from build123d import *

# Parameters (mm, degrees)
SKETCH41_R                  = 2.5527
BACK_PLATE_EXTRUDE_DEPTH    = 3.175
SKETCH71_W                  = 8.89
SKETCH71_H                  = 4.7625
SKETCH71_W_2                = 13.79855
SKETCH71_W_3                = 15.09395
BOSS_EXTRUDE26_DEPTH        = 3.175
SKETCH91_W                  = 4.9022
SKETCH91_H                  = 20.7645
SKETCH91_W_2                = 12.8524
SKETCH91_H_2                = 4.7625
SKETCH91_W_3                = 49.3649
SKETCH91_W_4                = 12.7762
BACK_PLATE_TOLERENCES_DEPTH = 4.175
SKETCH92_W                  = 2.794
SKETCH92_H                  = 26.9875
CUT_EXTRUDE1_DEPTH          = 4.175
FILLET27_R                  = 0.635
FILLET28_R                  = 0.635
SKETCH93_R                  = 0.635
CUT_EXTRUDE2_DEPTH          = 4.175
FILLET29_R                  = 0.635
FILLET29_OF_MIRROR26_R      = 0.635


with BuildPart() as part:
    # Sketch41 → Back Plate Extrude------------ (new body)
    with BuildSketch(Plane.XY.offset(152.527)):
        Polygon((-104.775, -7.9375), (-104.775, 12.7), (-109.5248, 12.7), (-109.5248, 3.175), (-112.395, 3.175), (-112.395, 25.4), (-104.775, 25.4), (104.775, 25.4), (112.395, 25.4), (112.395, 3.175), (109.5248, 3.175), (109.5248, 12.7), (104.775, 12.7), (104.775, -7.9375), align=None)
        with Locations((-100.0125, 3.9624)):
            Circle(SKETCH41_R, mode=Mode.SUBTRACT)
        with Locations((100.0125, 3.9624)):
            Circle(SKETCH41_R, mode=Mode.SUBTRACT)
        with Locations((23.8252, 20.6375)):
            Circle(SKETCH41_R, mode=Mode.SUBTRACT)
        with Locations((38.1127, 20.6375)):
            Circle(SKETCH41_R, mode=Mode.SUBTRACT)
        with Locations((52.4002, 20.6375)):
            Circle(SKETCH41_R, mode=Mode.SUBTRACT)
        with Locations((66.6877, 20.6375)):
            Circle(SKETCH41_R, mode=Mode.SUBTRACT)
        with Locations((-66.6877, 20.6375)):
            Circle(SKETCH41_R, mode=Mode.SUBTRACT)
        with Locations((-52.4002, 20.6375)):
            Circle(SKETCH41_R, mode=Mode.SUBTRACT)
        with Locations((-38.1127, 20.6375)):
            Circle(SKETCH41_R, mode=Mode.SUBTRACT)
        with Locations((-23.8252, 20.6375)):
            Circle(SKETCH41_R, mode=Mode.SUBTRACT)
        with Locations((-87.3125, 3.9624)):
            Circle(SKETCH41_R, mode=Mode.SUBTRACT)
        with Locations((87.3125, 3.9624)):
            Circle(SKETCH41_R, mode=Mode.SUBTRACT)
        with Locations((-63.5, -1.5875)):
            Circle(SKETCH41_R, mode=Mode.SUBTRACT)
        with Locations((63.5, -1.5875)):
            Circle(SKETCH41_R, mode=Mode.SUBTRACT)
    extrude(amount=BACK_PLATE_EXTRUDE_DEPTH)

    # Sketch71 → Boss-Extrude26 (add, through all)
    with BuildSketch(Plane.XY.offset(155.702)):
        with Locations((-107.95, 27.78125)):
            Rectangle(SKETCH71_W, SKETCH71_H)
        with Locations((-83.905725, 27.78125)):
            Rectangle(SKETCH71_W_2, SKETCH71_H)
        with Locations((-20.246975, 27.78125)):
            Rectangle(SKETCH71_W_3, SKETCH71_H)
    boss_extrude26 = extrude(amount=-BOSS_EXTRUDE26_DEPTH)

    # Mirror23: Boss-Extrude26 across plane
    add(boss_extrude26.mirror(Plane(origin=(0, 0, 0), x_dir=(0, 0, 1), z_dir=(1, 0, 0))))

    # Sketch91 → Back Plate Tolerences (cut, through all)
    with BuildSketch(Plane(origin=(0, 0, 152.527), x_dir=(-1, 0, 0), z_dir=(0, 0, -1))):
        with Locations((-107.1499, 2.44475)):
            Rectangle(SKETCH91_W, SKETCH91_H)
        with Locations((-97.155, 27.78125)):
            Rectangle(SKETCH91_W_2, SKETCH91_H_2)
        with Locations((-52.4002, 27.78125)):
            Rectangle(SKETCH91_W_3, SKETCH91_H_2)
        with Locations((-6.3881, 27.78125)):
            Rectangle(SKETCH91_W_4, SKETCH91_H_2)
    back_plate_tolerences = extrude(amount=-BACK_PLATE_TOLERENCES_DEPTH, mode=Mode.SUBTRACT)

    # Mirror25: Back Plate Tolerences across plane
    add(back_plate_tolerences.mirror(Plane(origin=(0, 0, 0), x_dir=(0, 0, 1), z_dir=(1, 0, 0))), mode=Mode.SUBTRACT)

    # Sketch92 → Cut-Extrude1 (cut, through all)
    with BuildSketch(Plane.XY.offset(155.702)):
        with Locations((-110.998, 16.66875)):
            Rectangle(SKETCH92_W, SKETCH92_H)
        with Locations((110.998, 16.66875)):
            Rectangle(SKETCH92_W, SKETCH92_H)
    extrude(amount=-CUT_EXTRUDE1_DEPTH, mode=Mode.SUBTRACT)

    # Fillet27
    fillet27_edges = [part.edges().sort_by_distance(p)[0] for p in [
        (104.6988, -7.9375, 154.1145),
        (109.601, 12.827, 154.1145),
        (-109.601, 12.827, 154.1145),
        (-104.6988, -7.9375, 154.1145),
        (-109.601, 30.1625, 154.1145),
        (109.601, 30.1625, 154.1145),
    ]]
    fillet(fillet27_edges, radius=FILLET27_R)

    # Fillet28
    fillet28_edges = [part.edges().sort_by_distance(p)[0] for p in [
        (103.5812, 30.1625, 154.1145),
        (90.7288, 30.1625, 154.1145),
        (77.08265, 30.1625, 154.1145),
        (27.71775, 30.1625, 154.1145),
        (12.7762, 30.1625, 154.1145),
        (-103.5812, 30.1625, 154.1145),
        (-90.7288, 30.1625, 154.1145),
        (-27.71775, 30.1625, 154.1145),
        (-77.08265, 30.1625, 154.1145),
        (-12.7762, 30.1625, 154.1145),
    ]]
    fillet(fillet28_edges, radius=FILLET28_R)

    # Sketch93 → Cut-Extrude2 (cut, through all)
    with BuildSketch(Plane.XY.offset(155.702)):
        with Locations((-104.6988, 12.827)):
            Circle(SKETCH93_R)
        with Locations((-103.5812, 25.4)):
            Circle(SKETCH93_R)
        with Locations((-90.7288, 25.4)):
            Circle(SKETCH93_R)
        with Locations((-77.08265, 25.4)):
            Circle(SKETCH93_R)
        with Locations((-27.71775, 25.4)):
            Circle(SKETCH93_R)
        with Locations((-12.7762, 25.4)):
            Circle(SKETCH93_R)
    cut_extrude2 = extrude(amount=-CUT_EXTRUDE2_DEPTH, mode=Mode.SUBTRACT)

    # Fillet29
    fillet29_edges = [part.edges().sort_by_distance(p)[0] for p in [
        (-105.3338, 12.827, 154.1145),
        (-103.5812, 26.035, 154.1145),
        (-27.71775, 26.035, 154.1145),
        (-12.7762, 26.035, 154.1145),
        (-90.7288, 26.035, 154.1145),
        (-77.08265, 26.035, 154.1145),
        (-104.6988, 12.192, 154.1145),
        (-102.9462, 25.4, 154.1145),
        (-91.3638, 25.4, 154.1145),
        (-76.44765, 25.4, 154.1145),
        (-28.35275, 25.4, 154.1145),
        (-12.1412, 25.4, 154.1145),
    ]]
    fillet(fillet29_edges, radius=FILLET29_R)

    # Mirror26: Cut-Extrude2 across plane
    add(cut_extrude2.mirror(Plane(origin=(0, 0, 0), x_dir=(0, 0, 1), z_dir=(1, 0, 0))), mode=Mode.SUBTRACT)

    # Fillet29 of Mirror26
    fillet29_of_mirror26_edges = [part.edges().sort_by_distance(p)[0] for p in [
        (105.3338, 12.827, 154.1145),
        (103.5812, 26.035, 154.1145),
        (27.71775, 26.035, 154.1145),
        (12.7762, 26.035, 154.1145),
        (90.7288, 26.035, 154.1145),
        (77.08265, 26.035, 154.1145),
        (104.6988, 12.192, 154.1145),
        (102.9462, 25.4, 154.1145),
        (91.3638, 25.4, 154.1145),
        (76.44765, 25.4, 154.1145),
        (28.35275, 25.4, 154.1145),
        (12.1412, 25.4, 154.1145),
    ]]
    fillet(fillet29_of_mirror26_edges, radius=FILLET29_OF_MIRROR26_R)


solid = part.part
Could you check a few things on this model? Use its own coordinates, in mm. Coordinates: 2 decimals unless noted, no trailing zeros. Order: outer loops, then holes, each group sorted by start corner. A loop starts at its lowest first (then second) coordinate and runs counter-clockwise, first axis right, second up. Notation, with made-up numbers: (47.25, 69.5) -> (91.25, 69.5) arc R24 cw to (91.25, 79.5) -> close; hole circle Ø7 at (66.5, 75.25). An arc over 180 degrees is marked (long way). One line per item, written item: value. Start each with the question number.
1) Imagine slicing it at A-A on x = 6.5. List the corners of the cut face in (y, z) for me.
2) If I drill on L1, parallel to X at y = 28, z = 153.7; L2, parallel to X at y = 3.5, z = 154.9; L3, parallel to X at y = 6, z = 153.2, over which ranges is the centre line in solid material (lowest first)? Write a range as [from, to].
3) We'd pull the mould along Y, two halves only. Please class faces 1 (the flat face through (2, 11, 152.527)), 2 (the cylindrical face through (49.85, 20.75, 154.09)): +Y half, -Y half, draft (parallel to the pull), parting line (faces both ways), or undercut.
4) I'm going to push flat-ended pins straight in: pin 1 (1 mm diameter, centred on x = 99.5, z = 154.5, fed in from +Y); pin 2 (1.5 mm diameter, centred on y = 6.5, z = 154.5, fed in from -X). Where does each tip first touch, or does it pass through?
Answer list:
1. outline: (-7.94, 152.53) -> (25.4, 152.53) -> (25.4, 155.7) -> (-7.94, 155.7) -> close
2. L1: x = [-109.6, -103.58], [-90.73, -77.08], [-27.72, -12.78], [12.78, 27.72], [77.08, 90.73], [103.58, 109.6]
2. L2: x = [-104.7, -102.52], [-97.5, -89.82], [-84.8, 84.8], [89.82, 97.5], [102.52, 104.7]
2. L3: x = [-104.7, -101.55], [-98.47, -88.85], [-85.77, 85.77], [88.85, 98.47], [101.55, 104.7]
3. face 1: draft
3. face 2: undercut
4. pin 1: stops at y = 25.4
4. pin 2: stops at x = -104.7
